The listing builds one solid part. Answer for the finished solid, in the listing's coordinates (mm). Coordinates: 2 decimals unless noted, no trailing zeros. Loops run counter-clockwise (first coordinate to the right, second up) from the corner with the lowest first, then second, coordinate; pieces in that order, holes last. Notation, with made-up numbers: (-36.5, 87) -> (20.5, 87) arc R19 ccw to (20.5, 93) -> close; hole circle Ø9 at (-18, 1.25). An arc over 180 degrees is marked (long way). Answer in a Markdown table with one row per item.
```python
from build123d import *

# Parameters (mm, degrees)
SKETCH1_R           = 4.953
BOSS_EXTRUDE1_DEPTH = 2.4384
SKETCH2_R           = 3.937
CUT_EXTRUDE1_DEPTH  = 2.4384
SKETCH3_R           = 0.508
BOSS_EXTRUDE2_DEPTH = 2.667
CUT_EXTRUDE2_START  = 3.747576
SKETCH4_R           = 1.2065
CUT_EXTRUDE2_DEPTH  = 1.205424
CIRPATTERN1_COUNT   = 7


with BuildPart() as part:
    # Sketch1 → Boss-Extrude1 (new body)
    with BuildSketch(Plane(origin=(0, 0, 0), x_dir=(1, 0, 0), z_dir=(0, 1, 0))):
        Circle(SKETCH1_R)
    extrude(amount=BOSS_EXTRUDE1_DEPTH)

    # Sketch2 → Cut-Extrude1 (cut)
    with BuildSketch(Plane(origin=(0, 2.4384, 0), x_dir=(1, 0, 0), z_dir=(0, 1, 0))):
        Circle(SKETCH2_R)
    extrude(amount=-CUT_EXTRUDE1_DEPTH, mode=Mode.SUBTRACT)

    # Sketch3 → Boss-Extrude2 (add)
    with BuildSketch(Plane(origin=(0, 0, 0), x_dir=(1, 0, 0), z_dir=(0, 1, 0))):
        with Locations((0, 4.445)):
            Circle(SKETCH3_R)
        with Locations((3.47524094, 2.771412169)):
            Circle(SKETCH3_R)
        with Locations((4.33355457, -0.989105551)):
            Circle(SKETCH3_R)
        with Locations((1.92861322, -4.004806618)):
            Circle(SKETCH3_R)
        with Locations((-1.92861322, -4.004806618)):
            Circle(SKETCH3_R)
        with Locations((-4.33355457, -0.989105551)):
            Circle(SKETCH3_R)
        with Locations((-3.47524094, 2.771412169)):
            Circle(SKETCH3_R)
    extrude(amount=BOSS_EXTRUDE2_DEPTH)

    # Sketch4 → Cut-Extrude2 (cut)
    with BuildSketch(Plane.XY.offset(CUT_EXTRUDE2_START)):
        with Locations((0, 1.8415)):
            Circle(SKETCH4_R)
    cut_extrude2 = extrude(amount=CUT_EXTRUDE2_DEPTH, mode=Mode.SUBTRACT)

    # CirPattern1: Cut-Extrude2 ×7 about axis
    cirpattern1_axis = Axis((0, 0, 0), (0, -1, 0))
    for i in range(1, CIRPATTERN1_COUNT):
        add(cut_extrude2.rotate(cirpattern1_axis, i * 360 / CIRPATTERN1_COUNT), mode=Mode.SUBTRACT)


solid = part.part
```
Item 1: A cutting plane is placed at B-B, the plane y = 2. Determine the outline of the cut face in (x, z), plus the area to 3 significant figures.
Findings below:
| item | result |
|---|---|
| outline | (-4.95, 0.1) -> (-3.92, 0.33) arc R3.94 cw to (-3.68, 1.4) -> (-4.5, 2.06) arc R4.95 ccw to start; (-4.42, -2.24) arc R4.95 ccw to (-3.16, -3.81) -> (-2.71, -2.86) arc R3.94 cw to (-3.39, -2) -> close; (-3.01, 3.93) -> (-2.19, 3.27) arc R3.94 cw to (-1.2, 3.75) -> (-1.2, 4.81) arc R4.95 ccw to start; (-1.01, -4.85) arc R4.95 ccw to (1.01, -4.85) -> (0.55, -3.9) arc R3.94 cw to (-0.55, -3.9) -> close; (1.2, 3.75) arc R3.94 cw to (2.19, 3.27) -> (3.01, 3.93) arc R4.95 ccw to (1.2, 4.81) -> close; (2.71, -2.86) -> (3.16, -3.81) arc R4.95 ccw to (4.42, -2.24) -> (3.39, -2) arc R3.94 cw to start; (3.68, 1.4) arc R3.94 cw to (3.92, 0.33) -> (4.95, 0.1) arc R4.95 ccw to (4.5, 2.06) -> close |
| area | 11.1 mm2 |
Item 2: Flat-ended cylindrical pins translate along their axes: pin 1 Ø1.5 at (y, z) = (2, 4) entering from +X; pin 2 Ø1 at (y, z) = (0.5, 1.5) entering from +X; pin 3 Ø1 at (x, z) = (3, 0.5) entering from +Y. Find the tip coordinate at first contact, or state that the pin passes through.
Findings below:
| item | result |
|---|---|
| pin 1 | stops at x = 3.13 |
| pin 2 | stops at x = 4.85 |
| pin 3 | passes through |
Item 3: Find the intervals of material crossed by probe 1 along X at (y, z) = (2.5, -2.75); probe 2 along X at (y, z) = (0.75, 0); probe 3 along Z at (x, y) = (-1.5, 0.2), in increasing order.
Findings below:
| item | result |
|---|---|
| probe 1 | x = -3.98 to -2.97, 2.97 to 3.98 |
| probe 2 | x = -4.95 to -3.94, 3.94 to 4.95 |
| probe 3 | z = -4.72 to -3.64, 3.64 to 4.72 |
Item 4: Determine the mould class of faces 1 (the face through (-0.7, 2.438, -4.4)), 2 (the face through (-0.035, 0.636, 4.342)) for opening direction X: +X half, -X half, draft (parallel to the pull), parting line (faces both ways), or undercut.
Findings below:
| item | result |
|---|---|
| face 1 | draft |
| face 2 | undercut |
Item 5: A cutting plane is placed at A-A, the plane y = 1.2. Determine the outline of the cut face in (x, z).
Findings below:
| item | result |
|---|---|
| outline | (-4.95, -0.08) -> (-3.93, 0.15) arc R3.94 cw to (-3.61, 1.57) -> (-4.43, 2.22) arc R4.95 ccw to start; (-4.5, -2.07) arc R4.95 ccw to (-3.02, -3.92) -> (-2.57, -2.98) arc R3.94 cw to (-3.48, -1.84) -> close; (-3.15, 3.82) -> (-2.34, 3.17) arc R3.94 cw to (-1.02, 3.8) -> (-1.02, 4.85) arc R4.95 ccw to start; (-1.18, -4.81) arc R4.95 ccw to (1.18, -4.81) -> (0.73, -3.87) arc R3.94 cw to (-0.73, -3.87) -> close; (1.02, 3.8) arc R3.94 cw to (2.34, 3.17) -> (3.15, 3.82) arc R4.95 ccw to (1.02, 4.85) -> close; (2.57, -2.98) -> (3.02, -3.92) arc R4.95 ccw to (4.5, -2.07) -> (3.48, -1.84) arc R3.94 cw to start; (3.61, 1.57) arc R3.94 cw to (3.93, 0.15) -> (4.95, -0.08) arc R4.95 ccw to (4.43, 2.22) -> close |
